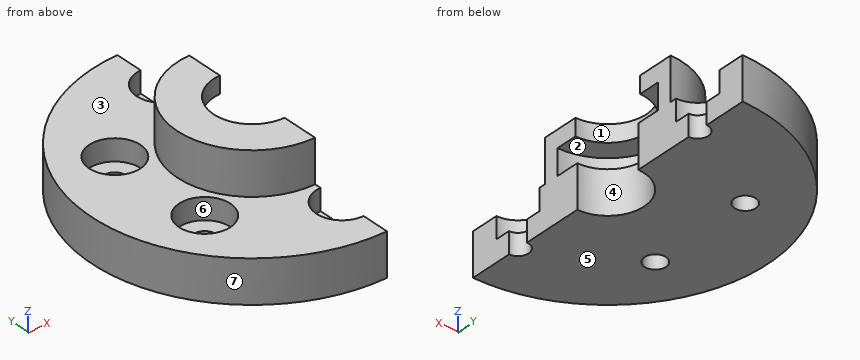
Autodesk Inventor part; units mm, degrees
ref_plane "YZ Plane" through (0, 0, 0) normal (1, 0, 0) x (0, 1, 0)
ref_plane "XZ Plane" through (0, 0, 0) normal (0, 1, 0) x (-1, 0, 0)
ref_plane "XY Plane" through (0, 0, 0) normal (0, 0, 1) x (1, 0, 0)
sketch "Sketch1" plane through (0, 0, 0) normal (0, 0, 1) x (1, 0, 0)
  circle A0 centre (0, 0) radius 37.5
  circle A1 centre (0, 25) radius 2.5
  circle A2 centre (0, 0) radius 25 construction
  circle A3 centre (-21.6506, 12.5) radius 2.5
  circle A4 centre (-21.6506, -12.5) radius 2.5
  circle A5 centre (0, -25) radius 2.5
  circle A6 centre (21.6506, -12.5) radius 2.5
  circle A7 centre (21.6506, 12.5) radius 2.5
  circle A8 centre (0, 0) radius 2.5
  dimension "d2" = 50
  dimension "d0" = 75
  dimension "d1" = 5
  dimension "d5" = 360
  dimension "d7" = 5
extrude "Extrusion1" add sketch "Sketch1" along normal blind 10
sketch "Sketch4" plane through (0, 0, 10) normal (0, 0, 1) x (1, 0, 0)
  circle A0 centre (0, 0) radius 2.5
  circle A1 centre (21.6506, 12.5) radius 2.5
  circle A2 centre (21.6506, -12.5) radius 2.5
  circle A3 centre (0, -25) radius 2.5
  circle A4 centre (-21.6506, -12.5) radius 2.5
  circle A5 centre (-21.6506, 12.5) radius 2.5
  circle A6 centre (0, 25) radius 2.5
  circle A7 centre (0, 0) radius 37.5
  circle A8 centre (0, 25) radius 6
  circle A9 centre (-21.6506, 12.5) radius 6
  circle A10 centre (-21.6506, -12.5) radius 6
  circle A11 centre (0, -25) radius 6
  circle A12 centre (21.6506, -12.5) radius 6
  circle A13 centre (21.6506, 12.5) radius 6
  dimension "d17" = 12
  dimension "d20" = 360
extrude "Extrusion4" cut sketch "Sketch4" against normal blind 5 contours A8 | A9 | A10 | A11 | A12 | A13
sketch "Sketch5" plane through (0, 0, 0) normal (0, 0, -1) x (-1, 0, 0)
  circle A0 centre (0, 0) radius 2.5
  circle A1 centre (0, 0) radius 8.5
  dimension "d24" = 17
extrude "Extrusion5" cut sketch "Sketch5" against normal blind 5
sketch "Sketch6" plane through (0, 0, 10) normal (0, 0, 1) x (1, 0, 0)
  circle A0 centre (0, 0) radius 2.5
  circle A1 centre (0, 0) radius 14
  circle A2 centre (0, 0) radius 17.5
  dimension "d35" = 35
  dimension "d36" = 28
extrude "Extrusion6" add sketch "Sketch6" along normal blind 10 contours A2
sketch "Sketch7" plane through (0, 0, 20) normal (0, 0, 1) x (1, 0, 0)
  circle A0 centre (0, 0) radius 9
  circle A1 centre (0, 0) radius 2.5
  circle A2 centre (0, 0) radius 17.5
  circle A3 centre (0, 0) radius 17.5
  dimension "d40" = 18
extrude "Extrusion7" add sketch "Sketch7" against normal blind 4 contours A2
sketch "Sketch8" plane through (0, 0, 20) normal (0, 0, 1) x (1, 0, 0)
  circle A0 centre (0, 0) radius 37.5
  line L0 (0, -37.5) -> (37.5, -37.5)
  line L1 (37.5, -37.5) -> (37.5, 37.5)
  line L2 (37.5, 37.5) -> (0, 37.5)
  line L3 (0, 37.5) -> (0, -37.5)
  point P0 (37.5, 0)
extrude "Extrusion8" cut sketch "Sketch8" against normal through all contours A0 L3 | L1 L0 A0 | A0 L2 L1 picked at (9.7729, 7.7936)
sketch "Sketch9" plane through (0, 0, 5) normal (0, 0, -1) x (-1, 0, 0)
  arc A0 (0, 14) -> (0, -14) centre (0, 0) ccw
  circle A1 centre (0, 0) radius 8.5 construction
  arc A2 (0, -14) -> (0, 14) centre (0, 0) ccw
  line L0 (0, 14) -> (-0.0015, 8.5)
  line L1 (0, -14) -> (0, -8.5)
  line L2 (0, -9) -> (0, -14)
  arc A3 (0, -8.5) -> (-0.0015, 8.5) centre (0, 0) ccw
  line L3 (0, 8.5) -> (0, 2.5)
  dimension "d39" = 17
extrude "Extrusion9" cut sketch "Sketch9" against normal blind 5 contours L0 A3 L1 A0
properties part number "BA008" material "ABS Plastic"
Source: CAD feature listing. Evaluate the final solid. Frame: model axes, mm. Face numbers are marked on the shaded views. A direction names the side the tool comes from. Coordinates: 2 decimals unless noted, no trailing zeros. Order: outer loops, then holes, each group sorted by start corner. A loop starts at its lowest first (then second) coordinate and runs counter-clockwise, first axis right, second up. Notation, with made-up numbers: (20, -30.5) - (36, -30.5) arc R31 cw to (36, 1.5) - close; hole circle Ø8 at (-38, -19.5). An arc over 180 degrees is marked (long way). One line per item, written item: value.
1) Ray query, line 1 (Z direction, x = -26.5, y = 18.5); line 2 (X direction, y = 16.5, z = 9); line 3 (Y direction, x = -2, z = 15.5). Return the intervals inside material, ascending. Write a range as [from, to].
Computed values:
line 1: z = [0, 10]
line 2: x = [-33.67, -26.12], [-17.18, 0]
line 3: y = [-17.39, -13.86], [13.86, 17.39]
2) Cut plane D-D on z = 3.5. Output: boundary loops of the cut face in (x, y).
Computed values:
outline: (0, -37.5) - (0, -27.5) arc R2.5 cw to (0, -22.5) - (0, -8.5) arc R8.5 cw to (0, 8.5) - (0, 22.5) arc R2.5 cw to (0, 27.5) - (0, 37.5) arc R37.5 ccw to start; hole circle Ø5 at (-21.65, -12.5); hole circle Ø5 at (-21.65, 12.5)
3) Reachability of the marked faces 1, 2 and 3 from +Z, -Z, +X, -X, +Y, -Y: full face, straight path, thin tool, end or side. Return the list, or none.
Computed values:
face 1: +Z, +X
face 2: +X
face 3: +Z, -X
4) Contact query for flat-ended pins moving along their axis: pin 1 (4 mm diameter, centred on x = -31.5, z = 11, fed in from +Y); pin 2 (6 mm diameter, centred on x = -16.5, y = -26.5, fed in from +Z); pin 3 (6 mm diameter, centred on x = -24.5, y = 12, fed in from +Z). Output: stop coordinate, or through.
Computed values:
pin 1: stops at y = 22.81
pin 2: stops at z = 10
pin 3: stops at z = 5
5) Mould query, pull axis Y, two halves, no side actions, for the marked faces 4, 5, 6 and 7. Classes: released by +Y, released by -Y, zero draft, split by the parting line, or undercut.
Computed values:
face 4: undercut
face 5: zero draft
face 6: undercut
face 7: split by the parting line
6) Cut plane C-C on y = -12.5. Output: boundary loops of the cut face in (x, z).
Computed values:
outline: (-35.36, 0) - (-24.15, 0) - (-24.15, 5) - (-27.65, 5) - (-27.65, 10) - (-35.36, 10) - close; (-19.15, 0) - (0, 0) - (0, 10) - (-6.3, 10) - (-6.3, 16) - (0, 16) - (0, 20) - (-12.25, 20) - (-12.25, 10) - (-15.65, 10) - (-15.65, 5) - (-19.15, 5) - close
7) Cut plane B-B on z = 7.5. Output: boundary loops of the cut face in (x, y), plus the area to 3 significant figures.
Computed values:
outline: (0, -37.5) - (0, -31) arc R6 cw to (0, -19) - (0, -8.5) arc R8.5 cw to (0, 8.5) - (0, 19) arc R6 cw to (0, 31) - (0, 37.5) arc R37.5 ccw to start; hole circle Ø12 at (-21.65, -12.5); hole circle Ø12 at (-21.65, 12.5)
area: 1,760 mm^2
8) Cut plane A-A on y = 0. Output: boundary loops of the cut face in (x, z), plus the area to 3 significant figures.
Computed values:
outline: (-37.5, 0) - (-8.5, 0) - (-8.5, 10) - (-14, 10) - (-14, 16) - (-9, 16) - (-9, 20) - (-17.5, 20) - (-17.5, 10) - (-37.5, 10) - close
area: 345 mm^2
